from build123d import *

# Parameters (mm, degrees)
F0_W     = 131.074406
F0_H     = 73.729352
F0_R     = 4.274249
F0_R_2   = 4.132324
F0_R_3   = 4.503614
F0_R_4   = 4.403148
F0_R_5   = 3.909793
F0_R_6   = 4.159305
F0_R_7   = 4.132325
F0_R_8   = 4.713948
F0_R_9   = 4.674234
F0_R_10  = 4.642219
F0_R_11  = 4.838842
F1_DEPTH = 25.4


with BuildPart() as f1:
    # F0 (on Front) → F1 (new body)
    with BuildSketch(Plane.XZ):
        with Locations((3.003787, -24.576451)):
            Rectangle(F0_W, F0_H)
        with Locations((-55.433549, -55.160478)):
            Circle(F0_R, mode=Mode.SUBTRACT)
        with Locations((-45.60297, -55.160478)):
            Circle(F0_R_2, mode=Mode.SUBTRACT)
        with Locations((-28.126383, -55.433549)):
            Circle(F0_R_3, mode=Mode.SUBTRACT)
        with Locations((-16.3843, -55.433549)):
            Circle(F0_R_4, mode=Mode.SUBTRACT)
        with Locations((-54.614335, 3.823003)):
            Circle(F0_R_5, mode=Mode.SUBTRACT)
        with Locations((-44.783756, 4.096075)):
            Circle(F0_R_6, mode=Mode.SUBTRACT)
        with Locations((-22.664949, 4.096075)):
            Circle(F0_R_7, mode=Mode.SUBTRACT)
        with Locations((-12.834369, 3.823003)):
            Circle(F0_R_2, mode=Mode.SUBTRACT)
        with Locations((43.964539, -6.553721)):
            Circle(F0_R_8, mode=Mode.SUBTRACT)
        with Locations((55.433553, -6.553721)):
            Circle(F0_R_9, mode=Mode.SUBTRACT)
        with Locations((43.964539, 5.188362)):
            Circle(F0_R_10, mode=Mode.SUBTRACT)
        with Locations((55.433553, 5.188362)):
            Circle(F0_R_11, mode=Mode.SUBTRACT)
    extrude(amount=F1_DEPTH)


solid = f1.part
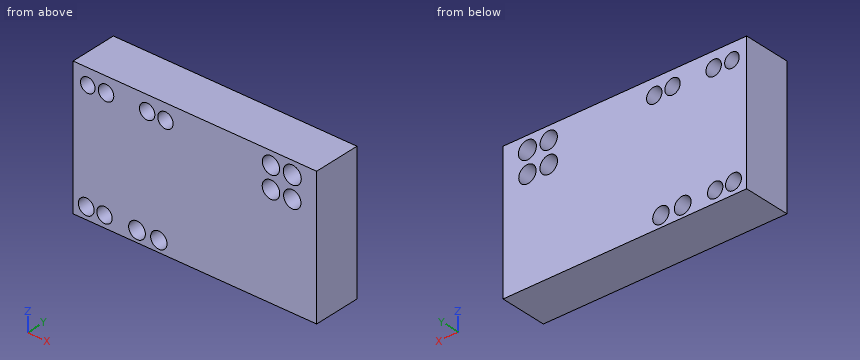
Verification items for the finished model (mm, model axes). Give positions to 0.01 mm unless a question says otherwise; leave off trailing zeros. Order: outer loops, then holes, each group sorted by start corner. A loop starts at its lowest first (then second) coordinate and runs counter-clockwise, first axis right, second up. Notation, with made-up numbers: M 80.5,22.5 L 115.5,22.5 A15 ccw 115.5,33.5 Z; hole C -24.75,-20.5 d1. An arc over 180 degrees is marked long. Answer as a JSON object with one key per item and string values. Group by question number.
1) Depth check by flat-ended pin: pin 1 Ø15 at (x, z) = (55.43, -6.55) entering from -Y; pin 2 Ø7.5 at (x, z) = (-22.66, 4.1) entering from +Y. Enter the tip coordinate at first touch or a pass-through.
2) Cross-section at B-B (x = 57). Enter the section's corners in (y, z).
3) Scan lines: line 1 along Z through (x, y) = (-55, -8.25); line 2 along X through (y, z) = (-20.75, -55.5); line 3 along Z through (x, y) = (-13, -19.75). Record each from-to range of solid material in increasing order. Write a range as [from, to].
4) Cross-section at D-D (y = -8.25). Give the number of separate pieces and of enclosed holes in the cut face, then the cut area to 3 significant figures.
5) Cross-section at A-A (z = 2). Enter the section's corners in (x, y).
6) Cross-section at C-C (z = -53). Enter the section's corners in (x, y).
Result sheet:
{
 "1": {"pin 1": "stops at y = -25.4", "pin 2": "passes through"},
 "2": {"outline": "M -25.4,-61.44 L 0,-61.44 L 0,-10.96 L -25.4,-10.96 Z; M -25.4,-2.15 L 0,-2.15 L 0,0.61 L -25.4,0.61 Z; M -25.4,9.77 L 0,9.77 L 0,12.29 L -25.4,12.29 Z"},
 "3": {"line 1": "z = [-61.44, -59.41], [-50.91, -0.07], [7.71, 12.29]", "line 2": "x = [-62.53, -59.69], [-51.17, -49.72], [-41.48, -32.63], [-23.62, -20.79], [-11.98, 68.54]", "line 3": "z = [-61.44, -58.25], [-52.62, -0.31], [7.95, 12.29]"},
 "4": {"separate pieces": "1", "enclosed holes": "12", "area": "8,940 mm2"},
 "5": {"outline": "M -62.53,-25.4 L -58.07,-25.4 L -58.07,0 L -62.53,0 Z; M -51.16,-25.4 L -48.38,-25.4 L -48.38,0 L -51.16,0 Z; M -41.19,-25.4 L -26.23,-25.4 L -26.23,0 L -41.19,0 Z; M -19.1,-25.4 L -16.54,-25.4 L -16.54,0 L -19.1,0 Z; M -9.13,-25.4 L 40.59,-25.4 L 40.59,0 L -9.13,0 Z; M 47.34,-25.4 L 51.79,-25.4 L 51.79,0 L 47.34,0 Z; M 59.07,-25.4 L 68.54,-25.4 L 68.54,0 L 59.07,0 Z"},
 "6": {"outline": "M -62.53,-25.4 L -59.12,-25.4 L -59.12,0 L -62.53,0 Z; M -51.75,-25.4 L -49.13,-25.4 L -49.13,0 L -51.75,0 Z; M -42.08,-25.4 L -31.92,-25.4 L -31.92,0 L -42.08,0 Z; M -24.34,-25.4 L -20.05,-25.4 L -20.05,0 L -24.34,0 Z; M -12.71,-25.4 L 68.54,-25.4 L 68.54,0 L -12.71,0 Z"}
}
